Geometry: final body of the model. Coordinates: model frame, mm. Coordinates: 2 decimals unless noted, no trailing zeros. Write each loop counter-clockwise with the first axis right and the second up, starting at its lowest first coordinate (ties: lowest second). Pieces come first, ordered by that corner, then holes. Notation, with made-up numbers: (89, -6) -> (116, -6) arc R25 cw to (116, 32) -> close; hole circle Ø1 at (-9.5, 81). An arc over 180 degrees is marked (long way). Answer as a JSON object with one key per item and string values. Group by question number.
```python
from build123d import *

# Parameters (mm, degrees)
SKETCH2_R           = 10.3
BOSS_EXTRUDE1_DEPTH = 29
SKETCH3_R           = 12.7
BOSS_EXTRUDE2_DEPTH = 2
CHAMFER1_SIZE       = 2


with BuildPart() as part:
    # Sketch2 → Boss-Extrude1 (new body)
    with BuildSketch(Plane.XY):
        with Locations(Location((0, 0, 0), (0, 0, 180))):
            Circle(SKETCH2_R)
    extrude(amount=BOSS_EXTRUDE1_DEPTH)

    # Sketch3 → Boss-Extrude2 (add)
    with BuildSketch(Plane.XY.offset(29)):
        Circle(SKETCH3_R)
    extrude(amount=BOSS_EXTRUDE2_DEPTH)

    # Chamfer1
    chamfer1_edges = [part.edges().sort_by_distance(p)[0] for p in [
        (-12.7, 0, 31),
    ]]
    chamfer(chamfer1_edges, length=CHAMFER1_SIZE - 0.0001)  # a hair under: the kernel refuses the full size


solid = part.part
```
Item 1: Contact query for flat-ended pins moving along their axis: pin 1 (1 mm diameter, centred on x = -0.5, y = -4.5, fed in from -Z); pin 2 (8 mm diameter, centred on y = 3.5, z = 9.5, fed in from +X); pin 3 (10 mm diameter, centred on x = -5.5, z = 17.5, fed in from -Y); pin 4 (5 mm diameter, centred on y = -8, z = 17, fed in from -X). Output: stop coordinate, or through.
Item 2: Mould query, pull axis Z, two halves, no side actions, for faces 1 (the flat face through (0, 0, 31)), 2 (the cylindrical face through (8.17, 6.27, 14.3)), 3 (the flat face through (-1, 10.41, 29)). Classes: +Z half, -Z half, draft (parallel to the pull), parting line (faces both ways), or undercut.
Item 3: Section D-D on z = 29.5. Output: boundary loops of the cut face in (x, y), then the cut area to 3 significant figures.
Item 4: Section C-C on z = 9. Output: boundary loops of the cut face in (x, y), then the cut area to 3 significant figures.
Item 5: Ray query, L1, parallel to Y at x = 1, z = 2.5; L2, parallel to X at y = -1.75, z = 4; L3, parallel to X at y = 3.5, z = 2. Return the intervals inside material, ascending. Write a range as [from, to].
Answer sheet:
{
 "1": {"pin 1": "stops at z = 0", "pin 2": "stops at x = 10.3", "pin 3": "stops at y = -10.29", "pin 4": "stops at x = -8.71"},
 "2": {"face 1": "+Z half", "face 2": "draft", "face 3": "-Z half"},
 "3": {"outline": "circle Ø24.4 at (0, 0)", "area": "468 mm^2"},
 "4": {"outline": "circle Ø20.6 at (0, 0)", "area": "333 mm^2"},
 "5": {"L1": "y = [-10.25, 10.25]", "L2": "x = [-10.15, 10.15]", "L3": "x = [-9.69, 9.69]"}
}
